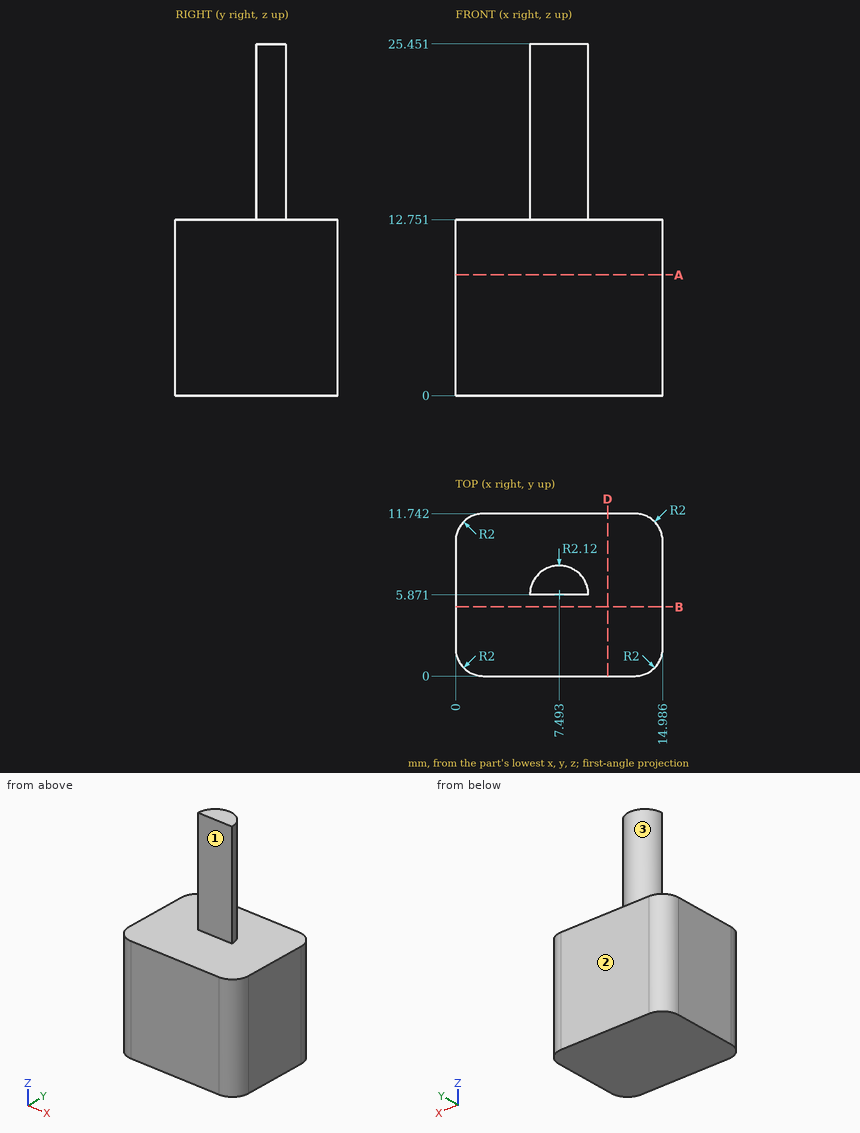
Can you work these out from the drawing? Everything is in mm from the part's minimum corner. A direction names the side the tool comes from. Coordinates: 2 decimals unless noted, no trailing zeros. Loops run counter-clockwise (first coordinate to the right, second up) from the corner with the lowest first, then second, coordinate; pieces in that order, holes last. Notation, with made-up numbers: (33.25, 46) -> (61.25, 46) arc R28 ccw to (61.25, 67) -> close; hole circle Ø2 at (27.25, 1.25). An arc over 180 degrees is marked (long way). Return JSON: item names as keys, results as strings.
1) Will these pins go through, and if not, where does the flat tip stop? pin 1 (6 mm diameter, centred on x = 9, z = 17.5, fed in from +Y); pin 2 (1.3 mm diameter, centred on x = 7.5, z = 17.5, fed in from -Y); pin 3 (3 mm diameter, centred on x = 3, y = 1.5, fed in from +Z); pin 4 (3 mm diameter, centred on x = 8, y = 5.5, fed in from -Z).
Results below:
{"pin 1": "y = 7.99", "pin 2": "y = 5.87", "pin 3": "z = 12.75", "pin 4": "z = 0"}
2) If we section it at B-B, the plane y = 5: Write out the boundary of the cut face in (x, z), then the cut area to 3 significant figures.
Results below:
{"outline": "(0, 0) -> (14.99, 0) -> (14.99, 12.75) -> (0, 12.75) -> close", "area": "191 mm²"}
3) I need wall thicknesses on line 1 (Z direction, x = 6.5, y = 8); line 2 (X direction, y = 1.25, z = 6.25) (1 decimal); line 3 (X direction, y = 10, z = 10.25). Which ranges of each line are inside material? Lowest first, please. Write a range as from..to.
Results below:
{"line 1": "0..12.75", "line 2": "0.1..14.8", "line 3": "0.02..14.97"}
4) For the marked faces 1, 2 and 3, which set-ups out of +Z, -Z, +X, -X, +Y, -Y let a thin tool reach every point of the face, with its end or its side?
Results below:
{"face 1": "+Z, +X, -X, -Y", "face 2": "+Z, -Z, +X, -X, +Y", "face 3": "+Z, +Y"}
5) If we section it at D-D, the plane x = 11: Write out the boundary of the cut face in (y, z).
Results below:
{"outline": "(0, 0) -> (11.74, 0) -> (11.74, 12.75) -> (0, 12.75) -> close"}
6) If we section it at A-A, the plane z = 8.75: Write out the boundary of the cut face in (x, y).
Results below:
{"outline": "(0, 2) arc R2 ccw to (2, 0) -> (12.99, 0) arc R2 ccw to (14.99, 2) -> (14.99, 9.74) arc R2 ccw to (12.99, 11.74) -> (2, 11.74) arc R2 ccw to (0, 9.74) -> close"}
